```python
from build123d import *

# Parameters (mm, degrees)
F0_W     = 12.7
F0_H     = 25.4
F1_DEPTH = 6.35
F2_R     = 5.08
F3_R     = 12.7
F5_DEPTH = 6.351


with BuildPart() as f1:
    # F0 (on Top) → F1 (new body)
    with BuildSketch(Plane.XY):
        with BuildLine():
            Line((-87.171328, 6.23762), (-74.471328, 6.23762))
            ThreePointArc((-74.471328, 6.23762), (-35.375303, 45.333645), (3.720721, 6.23762))
            Line((3.720721, 6.23762), (16.420721, 6.23762))
            ThreePointArc((16.420721, 6.23762), (1.250017, 42.862941), (-35.375303, 58.033645))
            Line((-35.375303, 58.033645), (-106.221328, 58.033645))
            Line((-106.221328, 58.033645), (-106.221328, 19.933645))
            Line((-106.221328, 19.933645), (-144.321328, 19.933645))
            Line((-144.321328, 19.933645), (-144.321328, 58.033645))
            Line((-144.321328, 58.033645), (-163.371328, 58.033645))
            Line((-163.371328, 58.033645), (-196.117352, 25.28762))
            Line((-196.117352, 25.28762), (-196.117352, 6.23762))
            Line((-196.117352, 6.23762), (-87.171328, 6.23762))
        make_face()
        with Locations((10.070721, -6.46238)):
            Rectangle(F0_W, F0_H)
    extrude(amount=F1_DEPTH)

    # F2
    f2_edges = [f1.edges().sort_by_distance(p)[0] for p in [
        (16.420721, -19.16238, 3.175),
        (3.720721, -19.16238, 3.175),
    ]]
    fillet(f2_edges, radius=F2_R)

    # F3
    f3_edges = [f1.edges().sort_by_distance(p)[0] for p in [
        (-74.471328, 6.23762, 3.175),
        (-196.117352, 25.28762, 3.175),
        (-163.371328, 58.033645, 3.175),
        (-196.117352, 6.23762, 3.175),
    ]]
    fillet(f3_edges, radius=F3_R)

    # F4 (on face) → F5 (cut, through all)
    with BuildSketch(Plane.XY.offset(6.35)):
        with BuildLine():
            ThreePointArc((-144.321328, 21.30846), (-144.42767, 20.911585), (-144.718203, 20.621053))
            ThreePointArc((-144.718203, 20.621053), (-144.882594, 19.372379), (-143.63392, 19.53677))
            ThreePointArc((-143.63392, 19.53677), (-143.343388, 19.827303), (-142.946513, 19.933645))
            Line((-142.946513, 19.933645), (-144.321328, 21.30846))
        make_face()
        with BuildLine():
            ThreePointArc((-105.824453, 20.621053), (-106.114986, 20.911585), (-106.221328, 21.30846))
            Line((-106.221328, 21.30846), (-107.596143, 19.933645))
            ThreePointArc((-107.596143, 19.933645), (-107.199268, 19.827303), (-106.908736, 19.53677))
            ThreePointArc((-106.908736, 19.53677), (-105.660062, 19.372379), (-105.824453, 20.621053))
        make_face()
    extrude(amount=-F5_DEPTH, mode=Mode.SUBTRACT)


solid = f1.part
```
For this review, take the finished solid that the model builds, in its own axes (mm). A direction names the side the tool comes from. Round coordinates to 2 decimals unless told otherwise and drop trailing zeros. Write each loop counter-clockwise with the first axis right and the second up, starting at its lowest first coordinate (ties: lowest second). Pieces come first, ordered by that corner, then holes. Notation, with made-up numbers: (38, 79) -> (60, 79) arc R30 cw to (60, 104) -> close; hole circle Ø7 at (60.25, -11.5). An arc over 180 degrees is marked (long way). One line per question, with ' | ' between items. Start each with the question number.
(1) Tool access review of faces 1 (the face through (-125, 19.934, 3)), 2 (the face through (-77.696, 8.989, 3.219)), 3 (the face through (-135, 6.238, 3)), 4 (the face through (-163.04, 57.04, 3.22)): name each direction out of +Z, -Z, +X, -X, +Y, -Y from which nothing blocks a thin tool from reaching the whole face with its end or side.
(2) Add section D-D, the plane y = -2.5. Write out the cut boundary in (x, z), plus the area to 3 significant figures.
(3) Add section B-B, the plane y = 27. Write out the cut boundary in (x, z), plus the area to 3 significant figures.
(4) Insertion check: P1, Ø1.9, axis at y = -3.5, z = 3.5, coming from the -X side; P2, Ø1.3, axis at x = -106.22, y = 19.93, coming from the -Z side; P3, Ø3, axis at y = 34.5, z = 1, coming from the +X side; P4, Ø1.9, axis at y = 41.5, z = 4, coming from the +X side. Each pin has a flat end and moves straight along its axis. Give the tip position at first contact, or say it passes through.
(5) Add section A-A, the plane z = 5.25. Write out the cut boundary in (x, y).
(6) For line 1 along X through (y, z) = (21.5, 3.25); line 2 along X through (y, z) = (36.5, 1.5); line 3 along Y through (x, z) = (-155, 3.5), list the stretches that pass through material, from the lowest coordinate up. Write a range as from..to.
(7) Add section C-C, the plane x = -127.5. Write out the cut boundary in (y, z), plus the area to 3 significant figures.
Answer list:
1) face 1: +Z, -Z, +Y | face 2: +Z, -Z, -Y | face 3: +Z, -Z, -X, -Y | face 4: +Z, -Z, -X, +Y
2) outline: (3.72, 0) -> (16.42, 0) -> (16.42, 6.35) -> (3.72, 6.35) -> close | area: 80.6 mm²
3) outline: (-194.03, 0) -> (-144.32, 0) -> (-144.32, 6.35) -> (-194.03, 6.35) -> close; (-106.22, 0) -> (-68.5, 0) -> (-68.5, 6.35) -> (-106.22, 6.35) -> close; (-2.25, 0) -> (12.08, 0) -> (12.08, 6.35) -> (-2.25, 6.35) -> close | area: 646 mm²
4) P1: x = 3.72 | P2: through | P3: x = 8.97 | P4: x = 3.43
5) outline: (-196.12, 18.94) arc R12.7 ccw to (-183.42, 6.24) -> (-85.59, 6.24) arc R12.7 ccw to (-73.28, 15.82) arc R39.1 cw to (3.72, 6.24) -> (3.72, -14.08) arc R5.08 ccw to (8.8, -19.16) -> (11.34, -19.16) arc R5.08 ccw to (16.42, -14.08) -> (16.42, 6.24) arc R51.8 ccw to (-35.38, 58.03) -> (-106.22, 58.03) -> (-106.22, 21.31) arc R0.79 ccw to (-105.82, 20.62) arc R0.79 cw (long way) to (-106.91, 19.54) arc R0.79 ccw to (-107.6, 19.93) -> (-142.95, 19.93) arc R0.79 ccw to (-143.63, 19.54) arc R0.79 cw (long way) to (-144.72, 20.62) arc R0.79 ccw to (-144.32, 21.31) -> (-144.32, 58.03) -> (-158.11, 58.03) arc R12.7 ccw to (-167.09, 54.31) -> (-192.4, 29.01) arc R12.7 ccw to (-196.12, 20.03) -> close
6) line 1: -196.03..-144.32, -106.22..-71.37, 0.62..14.12 | line 2: -184.9..-144.32, -106.22..-60.13, -10.62..6.66 | line 3: 6.24..58.03
7) outline: (6.24, 0) -> (19.93, 0) -> (19.93, 6.35) -> (6.24, 6.35) -> close | area: 87.0 mm²
